The drawing under review shows one solid part. Ordinate dimensions are in mm from its lowest x, y, z. A direction names the side the tool comes from. Round coordinates to 2 decimals unless told otherwise and drop trailing zeros. Write each loop counter-clockwise with the first axis right and the second up, starting at its lowest first coordinate (ties: lowest second). Pieces come first, ordered by that corner, then holes. Notation, with made-up numbers: M 7,62 L 24,62 A19 ccw 24,84 Z; hole C -0.75,-20.5 d9. An arc over 180 degrees is marked long. Write item = value, one per line. Start each with the question number.
Item 1: Take a section at D-D, the plane z = 89.5. Give the boundary of the cut face in (x, y).
Item 2: Take a section at A-A, the plane z = 60. Give the boundary of the cut face in (x, y).
Item 3: Take a section at C-C, the plane y = 87.5. Give the boundary of the cut face in (x, z), plus the area to 3 significant figures.
Item 4: To check wall thickness, follow line 1 along X through (y, z) = (131, 60); line 2 along Y through (x, z) = (72.5, 15); line 3 along Z through (x, y) = (91, 53). State the ranges of each line that lie inside material, in increasing order.
Item 5: For pin 1 Ø4 at (x, z) = (39.5, 92.5) entering from +Y; pin 2 Ø5 at (x, z) = (22, 32) entering from -Y; pin 3 Ø10 at (y, z) = (95.5, 24.5) entering from -X; pin 4 Ø5 at (x, y) = (65.5, 138) entering from +Z, all flat-tipped, find the tip position at first contact; note any pin that passes through.
Item 6: Tool access review of the marked faces 1, 2 and 3: name each direction out of +Z, -Z, +X, -X, +Y, -Y from which nothing blocks a thin tool from reaching the whole face with its end or side.
Item 7: Take a section at B-B, the plane x = 60. Give the boundary of the cut face in (y, z).
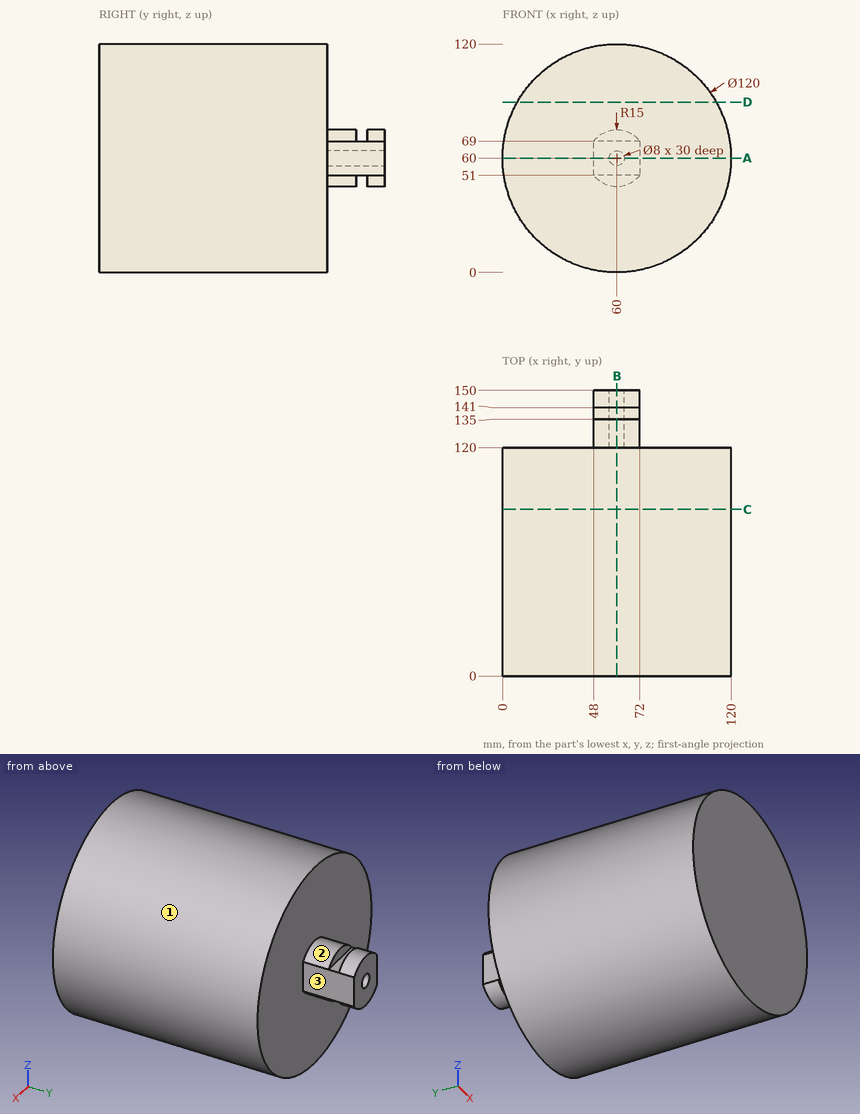
Response values:
q1.outline = M 7.75,0 L 112.25,0 L 112.25,120 L 7.75,120 Z
q2.outline = M 0,0 L 120,0 L 120,120 L 72,120 L 72,150 L 64,150 L 64,120 L 56,120 L 56,150 L 48,150 L 48,120 L 0,120 Z
q3.outline = C 60,60 d120
q3.area = 11,300 mm2
q4.line_1 = 48 to 56, 64 to 72
q4.line_2 = 0 to 120
q4.line_3 = 8.63 to 111.37
q5.pin_1 = 120
q5.pin_2 = 0
q5.pin_3 = 8.33
q5.pin_4 = 69
q6.face_1 = +Y, -Y
q6.face_2 = +Z, +Y
q6.face_3 = +Z, -Z, +X, +Y
q7.outline = M 0,0 L 120,0 L 120,45 L 135,45 L 135,51 L 141,51 L 141,45 L 150,45 L 150,56 L 120,56 L 120,64 L 150,64 L 150,75 L 141,75 L 141,69 L 135,69 L 135,75 L 120,75 L 120,120 L 0,120 Z
